Geometry: final body of the model. Coordinates: model frame, mm. Give positions to 0.01 mm unless a question says otherwise; leave off trailing zeros. Order: outer loops, then holes, each group sorted by start corner. A loop starts at its lowest first (then second) coordinate and runs counter-clockwise, first axis right, second up. Notation, with made-up numbers: M 69,25.25 L 100,25.25 A30 cw 100,57.25 Z; hole C 2,-18.5 d1. An arc over 180 degrees is marked long. Use CSV: the item, a comma, the result in double quotes.
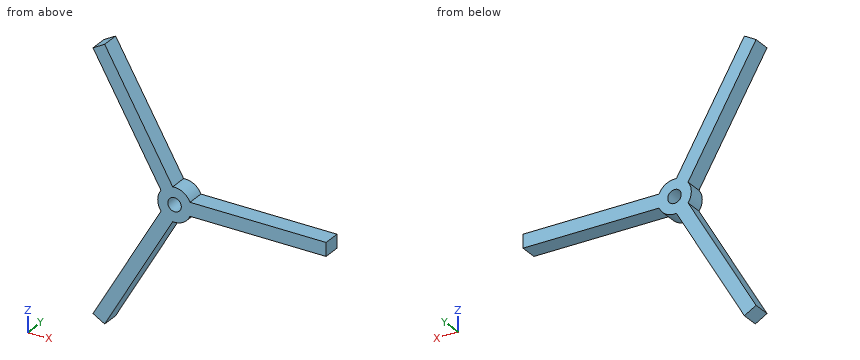
```python
from build123d import *

# Parameters (mm, degrees)
SKETCH1_R           = 6.35
SKETCH1_R_2         = 2.54
BOSS_EXTRUDE1_DEPTH = 6.604
BOSS_EXTRUDE2_START = -0.530129
SKETCH2_W           = 5.08
SKETCH2_H           = 6.604
BOSS_EXTRUDE2_DEPTH = 51.330129
CIRPATTERN1_COUNT   = 3


with BuildPart() as part:
    # Sketch1 → Boss-Extrude1 (new body)
    with BuildSketch(Plane(origin=(0, 0, 0), x_dir=(1, 0, 0), z_dir=(0, 1, 0))):
        Circle(SKETCH1_R)
        Circle(SKETCH1_R_2, mode=Mode.SUBTRACT)
    extrude(amount=BOSS_EXTRUDE1_DEPTH)

    # Sketch2 → Boss-Extrude2 (add)
    with BuildSketch(Plane(origin=(6.35, 0, 0), x_dir=(0, 0, -1), z_dir=(1, 0, 0)).offset(BOSS_EXTRUDE2_START)):
        with Locations((0, 3.302)):
            Rectangle(SKETCH2_W, SKETCH2_H)
    boss_extrude2 = extrude(amount=BOSS_EXTRUDE2_DEPTH)

    # CirPattern1: Boss-Extrude2 ×3 about axis
    cirpattern1_axis = Axis((0, 0, 0), (0, 1, 0))
    for i in range(1, CIRPATTERN1_COUNT):
        add(boss_extrude2.rotate(cirpattern1_axis, i * 360 / CIRPATTERN1_COUNT))


solid = part.part
```
1. Section C-C, the plane x = 39.5. Return the cut outline in (y, z), plus the area to 3 significant figures.
Answer:
outline,"M 0,-2.54 L 6.6,-2.54 L 6.6,2.54 L 0,2.54 Z"
area,"33.5 mm2"
2. Section A-A, the plane z = 0. Return the cut outline in (x, y).
Answer:
outline,"M -6.35,0 L -2.54,0 L -2.54,6.6 L -6.35,6.6 Z; M 2.54,0 L 57.15,0 L 57.15,6.6 L 2.54,6.6 Z"
3. Section D-D, the plane x = 4. Return the cut outline in (y, z).
Answer:
outline,"M 0,-4.93 L 6.6,-4.93 L 6.6,4.93 L 0,4.93 Z"
4. Pin query (flat end, axial travel): pin 1 Ø1.5 at (y, z) = (5, -18.5) entering from -X; pin 2 Ø1.5 at (x, y) = (-14.5, 4.5) entering from -Z; pin 3 Ø2 at (x, y) = (27, 1.5) entering from -Z. Return the tip coordinate at first contact, or that it passes through.
Answer:
pin 1,"x = -14.05"
pin 2,"z = -31.49"
pin 3,"z = -2.54"
5. Section B-B, the plane y = 4. Return the cut outline in (x, z).
Answer:
outline,"M -30.77,-48.22 L -26.38,-50.76 L -0.71,-6.31 A6.35 ccw 5.82,-2.54 L 57.15,-2.54 L 57.15,2.54 L 5.82,2.54 A6.35 ccw -0.71,6.31 L -26.38,50.76 L -30.77,48.22 L -5.11,3.77 A6.35 ccw -5.11,-3.77 Z; hole C 0,0 d5.08"
6. Line query: line 1 (X direction, y = 4, z = 0); line 2 (Z direction, x = 0, y = 3); line 3 (X direction, y = 3.75, z = 1.5). Output: solid intervals per line, ascending.
Answer:
line 1,"-6.35 to -2.54, 2.54 to 57.15"
line 2,"-6.35 to -2.54, 2.54 to 6.35"
line 3,"-6.17 to -2.05, 2.05 to 57.15"
